Can you work these out from the model? Positions are in its coordinate system, mm. Face numbers are marked on the shaded views. A direction names the side the tool comes from. Round coordinates to 2 decimals unless told otherwise and drop trailing zeros. Write each loop counter-clockwise with the first axis right and the second up, starting at its lowest first coordinate (ties: lowest second). Pieces come first, ordered by that corner, then holes. Notation, with made-up numbers: M -39.75,34.25 L 2.25,34.25 A27 ccw 2.25,72.25 Z; hole C 80.25,47 d4. An arc over 180 degrees is marked long. Answer as a JSON object with one key per item and string values. Group by question number.
1) Suppose I cut it at A-A, the plane x = 0. Write out the boundary of the cut face in (y, z).
2) Please list where these lines run through material, in increasing order: L1, parallel to Y at x = 8.5, z = -27.5; L2, parallel to Y at x = 6.5, z = -18; L3, parallel to Z at x = 19, y = -8. Write a range as [from, to].
3) I'm going to push flat-ended pins straight in: pin 1 Ø8 at (x, y) = (-2.5, -24.5) entering from -Z; pin 2 Ø8 at (x, y) = (28, -11) entering from +Z; pin 3 Ø5 at (x, z) = (20.5, 17.5) entering from +Y; pin 4 Ø1 at (y, z) = (-38.5, -29) entering from -X. Where does each tip first touch, or does it pass through?
4) Suppose I cut it at C-C, the plane y = -40. Write out the boundary of the cut face in (x, z), and give its area (3 significant figures).
5) Suppose I cut it at B-B, the plane z = 0. Write out the boundary of the cut face in (x, y).
6) On a 3-axis mill with a long thin cutter (end or side, diameter ignored), from which of +Z, -Z, +X, -X, +Y, -Y can I reach the whole of each face in a straight line? I mean the marked faces 1 and 2. Say none if no direction works.
from build123d import *

# Parameters (mm, degrees)
F0_R     = 37.5
F1_DEPTH = 50
F2_R     = 24.069175
F3_DEPTH = 10
F4_R     = 5.08
F5_R     = 5.08


with BuildPart() as f1:
    # F0 (on Front) → F1 (new body)
    with BuildSketch(Plane.XZ):
        Circle(F0_R)
    extrude(amount=F1_DEPTH)

    # F2 (on face) → F3 (join)
    with BuildSketch(Plane.XZ.offset(50)):
        Circle(F2_R)
    extrude(amount=F3_DEPTH)

    # F4
    f4_edges = [f1.edges().sort_by_distance(p)[0] for p in [
        (37.5, -25, 0),
        (-37.5, 0, 0),
        (-37.5, -50, 0),
    ]]
    fillet(f4_edges, radius=F4_R)

    # F5
    f5_edges = [f1.edges().sort_by_distance(p)[0] for p in [
        (-24.069175, -60, 0),
    ]]
    fillet(f5_edges, radius=F5_R)


solid = f1.part
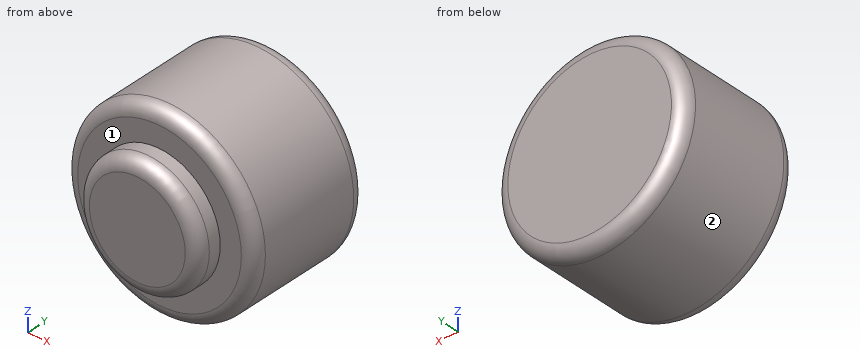
Results:
{
 "1": {"outline": "M -60,-18.99 A5.08 ccw -54.92,-24.07 L -50,-24.07 L -50,-32.42 A5.08 ccw -44.92,-37.5 L -5.08,-37.5 A5.08 ccw 0,-32.42 L 0,32.42 A5.08 ccw -5.08,37.5 L -44.92,37.5 A5.08 ccw -50,32.42 L -50,24.07 L -54.92,24.07 A5.08 ccw -60,18.99 Z"},
 "2": {"L1": "[-50, 0]", "L2": "[-60, 0]", "L3": "[-32.33, 32.33]"},
 "3": {"pin 1": "z = -37.5", "pin 2": "z = 28.81", "pin 3": "y = 0", "pin 4": "x = -24.37"},
 "4": {"outline": "C 0,0 d75", "area": "4,420 mm^2"},
 "5": {"outline": "M -37.5,-44.92 A5.08 ccw -32.42,-50 L -24.07,-50 L -24.07,-54.92 A5.08 ccw -18.99,-60 L 18.99,-60 A5.08 ccw 24.07,-54.92 L 24.07,-50 L 32.42,-50 A5.08 ccw 37.5,-44.92 L 37.5,-5.08 A5.08 ccw 32.42,0 L -32.42,0 A5.08 ccw -37.5,-5.08 Z"},
 "6": {"face 1": "-Y", "face 2": "+Y, -Y"}
}
